Verification items for this drawing (mm, ordinates from the low corner). A direction names the side the tool comes from. Coordinates: 2 decimals unless noted, no trailing zeros. Order: outer loops, then holes, each group sorted by start corner. A loop starts at its lowest first (then second) coordinate and runs counter-clockwise, first axis right, second up. Notation, with made-up numbers: M -12.75,67 L 13.25,67 A30 ccw 13.25,92 Z; hole C -14,88.25 d9. An arc over 180 degrees is marked long. Return JSON: item names as keys, results as strings. Group by question number.
1. Section check D-D, the plane y = 30. Record the cut outline in (x, z), plus the area to 3 significant figures.
2. Gauge pin test, flat ends, axial feed: pin 1 (14 mm diameter, centred on y = 33, z = 15, fed in from +X); pin 2 (5 mm diameter, centred on y = 46.15, z = 8.85, fed in from -X); pin 3 (1 mm diameter, centred on x = 9.5, z = 11, fed in from +Y). Record the tip position at first contact, or that the pin passes through.
3. Section check A-A, the plane y = 46.15. Record the cut outline in (x, z).
4. Set-up check for the marked faces 1 and 2: record each of +Z, -Z, +X, -X, +Y, -Y from which the full face is reachable in a straight line by a thin tool's end or side.
5. Section check C-C, the plane z = 25. Record the cut outline in (x, y).
6. Material ranges on line 1 along Y through (x, z) = (2.3, 41.15); line 2 along Y through (x, z) = (1, 41); line 3 along Z through (x, y) = (2, 13), recorded low to high.
7. Section check B-B, the plane x = 27. Record the cut outline in (y, z).
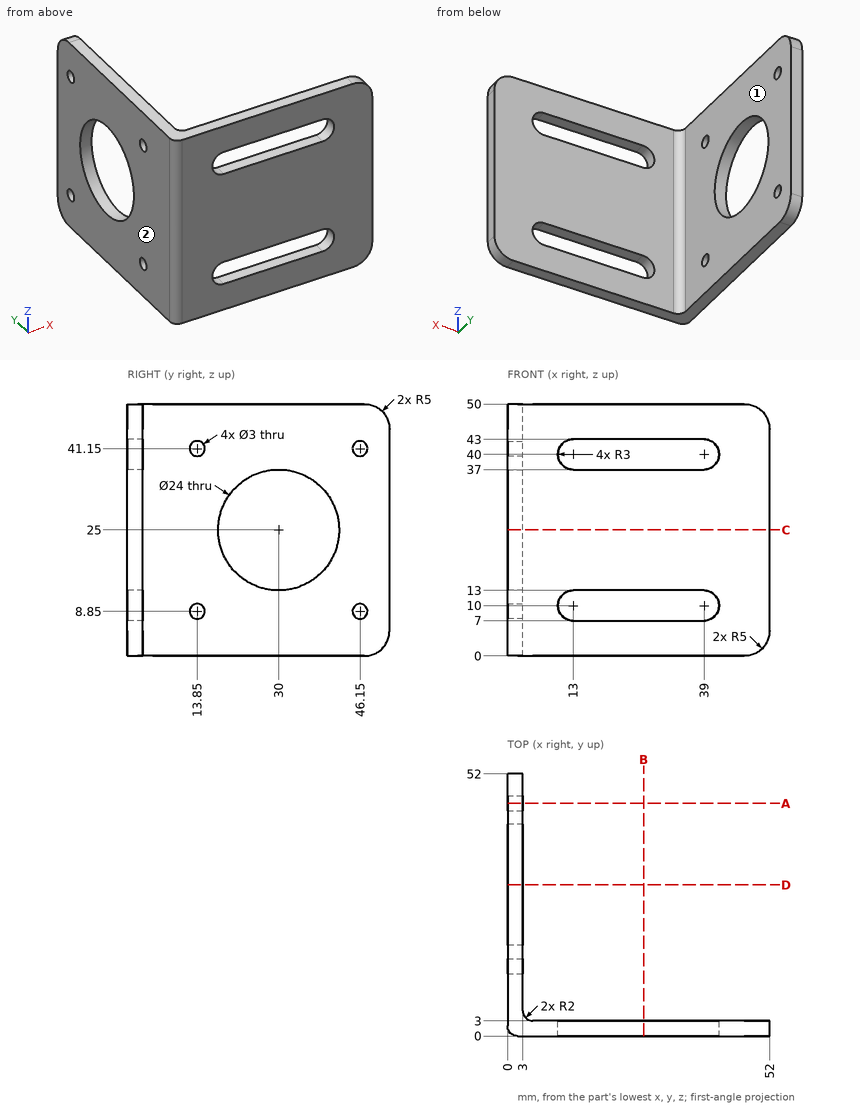
Answers follow:
{
 "1": {"outline": "M 0,0 L 3,0 L 3,13 L 0,13 Z; M 0,37 L 3,37 L 3,50 L 0,50 Z", "area": "78.0 mm^2"},
 "2": {"pin 1": "x = 3", "pin 2": "x = 0", "pin 3": "y = 3"},
 "3": {"outline": "M 0,0 L 3,0 L 3,7.35 L 0,7.35 Z; M 0,10.35 L 3,10.35 L 3,39.65 L 0,39.65 Z; M 0,42.65 L 3,42.65 L 3,50 L 0,50 Z"},
 "4": {"face 1": "+Z, -Z, +X, +Y", "face 2": "+Z, -Z, -X, +Y, -Y"},
 "5": {"outline": "M 0,2 A2 ccw 2,0 L 52,0 L 52,3 L 5,3 A2 cw 3,5 L 3,18 L 0,18 Z; M 0,42 L 3,42 L 3,52 L 0,52 Z"},
 "6": {"line 1": "0 to 12.35, 15.35 to 44.65, 47.65 to 52", "line 2": "0.27 to 12.36, 15.34 to 44.66, 47.64 to 52", "line 3": "0 to 7.61, 10.09 to 39.91, 42.39 to 50"},
 "7": {"outline": "M 0,0 L 3,0 L 3,7 L 0,7 Z; M 0,13 L 3,13 L 3,37 L 0,37 Z; M 0,43 L 3,43 L 3,50 L 0,50 Z"}
}
